Check sheet for the modelled part. Datum: model origin and axes. Units: mm. A direction names the side the tool comes from. Give positions to 0.01 mm unless a question says otherwise; leave off trailing zeros. Order: outer loops, then holes, each group sorted by start corner. A loop starts at its lowest first (then second) coordinate and runs counter-clockwise, first axis right, second up.
from build123d import *

# Parameters (mm, degrees)
BOSS_EXTRUDE1_DEPTH = 20
SKETCH2_R           = 4
CUT_EXTRUDE2_DEPTH  = 8
CUT_EXTRUDE4_DEPTH  = 10
SKETCH4_R           = 2.6
CUT_EXTRUDE5_DEPTH  = 1.5


with BuildPart() as part:
    # Sketch1 → Boss-Extrude1 (new body)
    with BuildSketch(Plane(origin=(0, 0, 0), x_dir=(1, 0, 0), z_dir=(0, 1, 0))):
        with BuildLine():
            Line((-41.301242739, 22.74889672), (-43.801242739, 22.74889672))
            Line((-43.801242739, 22.74889672), (-43.801242739, 10.24889672))
            ThreePointArc((-43.801242739, 10.24889672), (-52.640077504, 31.587731485), (-31.301242739, 22.74889672))
            Line((-31.301242739, 22.74889672), (-31.301242739, -37.25110328))
            Line((-31.301242739, -37.25110328), (-21.301242739, -37.25110328))
            Line((-21.301242739, -37.25110328), (-21.301242739, 22.74889672))
            Line((-21.301242739, 22.74889672), (-26.392335279, 22.74889672))
            ThreePointArc((-26.392335279, 22.74889672), (-56.111199256, 35.058853238), (-43.801242739, 5.339989261))
            Line((-43.801242739, 5.339989261), (-43.801242739, -37.25110328))
            Line((-43.801242739, -37.25110328), (-41.301242739, -37.25110328))
            Line((-41.301242739, -37.25110328), (-41.301242739, 22.74889672))
        make_face()
    extrude(amount=BOSS_EXTRUDE1_DEPTH)

    # Sketch2 → Cut-Extrude2 (cut)
    with BuildSketch(Plane.ZY.offset(31.301242739)):
        with Locations((17.25110328, 10)):
            Circle(SKETCH2_R)
    extrude(amount=-CUT_EXTRUDE2_DEPTH, mode=Mode.SUBTRACT)

    # Sketch3 → Cut-Extrude4 (cut)
    with BuildSketch(Plane(origin=(-21.301242739, 0, 0), x_dir=(0, 0, -1), z_dir=(1, 0, 0))):
        Polygon((-24.75110328, 10), (-27.75110328, 10.5), (-27.75110328, 9.5), align=None)
        Polygon((-21.75110328, 10.5), (-27.75110328, 10.5), (-24.75110328, 10), align=None)
        Polygon((-21.75110328, 10.5), (-24.75110328, 10), (-21.75110328, 9.5), align=None)
        Polygon((-21.75110328, 9.5), (-24.75110328, 10), (-27.75110328, 9.5), align=None)
        Polygon((-17.25110328, 10), (-20.25110328, 10.5), (-20.25110328, 9.5), align=None)
        Polygon((-14.25110328, 10.5), (-17.25110328, 10), (-14.25110328, 9.5), align=None)
        Polygon((-14.25110328, 10.5), (-20.25110328, 10.5), (-17.25110328, 10), align=None)
        Polygon((-14.25110328, 9.5), (-17.25110328, 10), (-20.25110328, 9.5), align=None)
    extrude(amount=-CUT_EXTRUDE4_DEPTH, mode=Mode.SUBTRACT)

    # Sketch4 → Cut-Extrude5 (cut)
    with BuildSketch(Plane.ZY.offset(31.301242739)):
        with Locations((24.75110328, 10)):
            Circle(SKETCH4_R)
    extrude(amount=-CUT_EXTRUDE5_DEPTH, mode=Mode.SUBTRACT)


solid = part.part
1) Section check C-C, the plane z = 17. Record the cut outline in (x, y), then the cut area to 3 significant figures.
Recorded:
outline: (-43.8, 0) - (-41.3, 0) - (-41.3, 20) - (-43.8, 20) - close; (-31.3, 0) - (-21.3, 0) - (-21.3, 9.5) - (-23.3, 9.5) - (-23.3, 6.01) - (-31.3, 6.01) - close; (-31.3, 13.99) - (-23.3, 13.99) - (-23.3, 10.5) - (-21.3, 10.5) - (-21.3, 20) - (-31.3, 20) - close
area: 184 mm2
2) Material ranges on L1, parallel to X at y = 8.5, z = 10.5; L2, parallel to Y at x = -26, z = 27; L3, parallel to Z at x = -44, y = 15.75, recorded low to high.
Recorded:
L1: x = -43.8 to -41.3, -31.3 to -21.3
L2: y = 0 to 9.5, 10.5 to 20
L3: z = -40.16 to -35.25, -10.25 to -5.34
3) Section check D-D, the plane z = -27. Record the cut outline in (x, y).
Recorded:
outline: (-60.68, 0) - (-55.56, 0) - (-55.56, 20) - (-60.68, 20) - close; (-32.05, 0) - (-26.92, 0) - (-26.92, 20) - (-32.05, 20) - close
4) Section check B-B, the plane z = -16. Record the cut outline in (x, y), then the cut area to 3 significant figures.
Recorded:
outline: (-59.85, 0) - (-54.32, 0) - (-54.32, 20) - (-59.85, 20) - close; (-43.8, 0) - (-41.3, 0) - (-41.3, 20) - (-43.8, 20) - close; (-31.3, 0) - (-21.3, 0) - (-21.3, 20) - (-31.3, 20) - close
area: 361 mm2
5) Set-up check for faces 4 (the face through (-31.301, 10, 7)), 5 (the face through (-27.357, 13.966, 16.73)), 6 (the face through (-22, 9.5, 17)): record each of +Z, -Z, +X, -X, +Y, -Y from which the full face is reachable in a straight line by a thin tool's end or side.
Recorded:
face 4: +Z, +Y, -Y
face 5: none
face 6: +X
6) Depth check by flat-ended pin: pin 1 Ø8 at (x, y) = (-55, 8.5) entering from +Z; pin 2 Ø5 at (x, y) = (-40, 16) entering from +Z; pin 3 Ø3 at (x, y) = (-47.5, 8.5) entering from +Z; pin 4 Ø5.5 at (x, y) = (-23, 8) entering from -Z. Enter the tip coordinate at first touch or a pass-through.
Recorded:
pin 1: stops at z = -6.9
pin 2: stops at z = 37.25
pin 3: stops at z = -5.48
pin 4: stops at z = -22.75
7) Draft check along Z on faces 1 (the face through (-30.6, 12.6, 24.8)), 2 (the face through (-43, 10, 37.251)), 3 (the face through (-55.699, 9.86, -35.458)). Enter one of: +Z half, -Z half, draft (parallel to the pull), parting line (faces both ways), or undercut.
Recorded:
face 1: undercut
face 2: +Z half
face 3: parting line
8) Section check A-A, the plane z = 30.5. Record the cut outline in (x, y), then the cut area to 3 significant figures.
Recorded:
outline: (-43.8, 0) - (-41.3, 0) - (-41.3, 20) - (-43.8, 20) - close; (-31.3, 0) - (-21.3, 0) - (-21.3, 20) - (-31.3, 20) - close
area: 250 mm2
